from build123d import *

# Parameters (mm, degrees)
CUBE001_W     = 16
CUBE001_H     = 300
CUBE001_DEPTH = 810
CUBE002_W     = 590
CUBE002_H     = 300
CUBE002_DEPTH = 16
CUBE003_W     = 590
CUBE003_H     = 300
CUBE003_DEPTH = 789
CUBE_W        = 16
CUBE_H        = 300
CUBE_DEPTH    = 810


with BuildPart() as cube001:
    # cube001 → cube001 (new body)
    with BuildSketch(Plane(origin=(606, 0, 0), x_dir=(1, 0, 0), z_dir=(0, 0, 1))):
        with Locations((8, 150)):
            Rectangle(CUBE001_W, CUBE001_H)
    extrude(amount=CUBE001_DEPTH)


with BuildPart() as cube002:
    # cube002 → cube002 (new body)
    with BuildSketch(Plane(origin=(16, 0, 789), x_dir=(1, 0, 0), z_dir=(0, 0, 1))):
        with Locations((295, 150)):
            Rectangle(CUBE002_W, CUBE002_H)
    extrude(amount=CUBE002_DEPTH)


with BuildPart() as cube003:
    # cube003 → cube003 (new body)
    with BuildSketch(Plane(origin=(16, 0, 0), x_dir=(1, 0, 0), z_dir=(0, 0, 1))):
        with Locations((295, 150)):
            Rectangle(CUBE003_W, CUBE003_H)
    extrude(amount=CUBE003_DEPTH)


with BuildPart() as base_drawers:
    # cube → cube (new body)
    with BuildSketch(Plane.XY):
        with Locations((8, 150)):
            Rectangle(CUBE_W, CUBE_H)
    extrude(amount=CUBE_DEPTH)

    # Group: union cube001, cube002, cube003
    add(cube001.part)
    add(cube002.part)
    add(cube003.part)


solid = base_drawers.part
Geometry: final body of the model. Coordinates: model frame, mm. Give positions to 0.01 mm unless a question says otherwise; leave off trailing zeros. Return JSON: item names as keys, results as strings. Group by question number.
1) First-contact query: P1, Ø5, axis at x = 436, y = 117.5, coming from the +Z side. Flat tip, straight axial feed; report the tip coordinate or a pass-through.
2) Line query: line 1 (Z direction, x = 34.5, y = 66). Output: solid intervals per line, ascending.
3) Mould query, pull axis X, two halves, no side actions, for faces 1 (the flat face through (614, 152, 810)), 2 (the flat face through (307, 152, 805)), 3 (the flat face through (622, 148, 399)), 4 (the flat face through (0, 148, 399)). Classes: released by +X, released by -X, zero draft, split by the parting line, or undercut.
Filled in:
{
 "1": {"P1": "stops at z = 805"},
 "2": {"line 1": "z = 0 to 805"},
 "3": {"face 1": "zero draft", "face 2": "undercut", "face 3": "released by +X", "face 4": "released by -X"}
}
